Autodesk Inventor part; units mm, degrees
ref_plane "Work Plane1" through (-106.5, -37, 0) normal (1, 0, 0) x (0, 1, 0)
ref_plane "Work Plane2" through (-183, -37, 0) normal (1, 0, 0) x (0, 1, 0)
ref_plane "Work Plane3" through (-106.5, -37, -17.5) normal (0, -1, 0) x (1, 0, 0)
sketch "Sketch1" plane through (0, 0, 0) normal (0, 0, 1) x (1, 0, 0)
  line L0 (-183, -19.5) -> (-106.5, -19.5)
  line L1 (-106.5, -19.5) -> (-106.5, -54.5)
  line L2 (-106.5, -54.5) -> (-183, -54.5)
  line L3 (-183, -54.5) -> (-183, -19.5)
  line L4 (-194, -37) -> (-96, -37) construction
  line L5 (-183, -22) -> (-157.5, -22)
  line L6 (-157.5, -22) -> (-157.5, -37)
  line L7 (-157.5, -24.5) -> (-116.5, -24.5)
  line L8 (-116.5, -37) -> (-116.5, -22)
  line L9 (-116.5, -22) -> (-106.5, -22)
  line L10 (-183, -52) -> (-157.5, -52) construction
  line L11 (-157.5, -52) -> (-157.5, -37) construction
  line L12 (-157.5, -49.5) -> (-116.5, -49.5) construction
  line L13 (-116.5, -37) -> (-116.5, -52) construction
  line L14 (-116.5, -52) -> (-106.5, -52) construction
  line L15 (-183, -37) -> (-106.5, -37)
  point P0 (0, 0)
  dimension "d0" = 76.5
  dimension "d1" = 35
  dimension "d2" = 30
  dimension "d3" = 25.5
  dimension "d4" = 10
  dimension "d5" = 25
  dimension "d6" = 30
sketch "Sketch3" plane through (0, 0, 0) normal (1, 0, 0) x (0, 1, 0)
  point P0 (0, 0)
ref_plane "Work Plane1" through (-106.5, -37, 0) normal (1, 0, 0) x (0, 1, 0)
sketch "Sketch4" plane through (-106.5, -37, 0) normal (1, 0, 0) x (0, 1, 0)
  point P0 (37, 0)
sketch "Sketch5" plane through (-106.5, -37, 0) normal (1, 0, 0) x (0, 1, 0)
  line L0 (-17.5, 17.5) -> (17.5, 17.5)
  line L1 (17.5, 17.5) -> (17.5, -17.5)
  line L2 (17.5, -17.5) -> (-17.5, -17.5)
  line L3 (-17.5, -17.5) -> (-17.5, 17.5)
  line L4 (-17.5, 17.5) -> (17.5, -17.5) construction
  line L5 (17.5, 17.5) -> (-17.5, -17.5) construction
  point P0 (37, 0)
  point P1 (0, 0)
  dimension "d10" = 35
  dimension "d11" = 35
ref_plane "Work Plane2" through (-183, -37, 0) normal (1, 0, 0) x (0, 1, 0)
extrude "Extrusion1" add sketch "Sketch5" against normal up to surface (76.5 mm away)
revolve "Revolution2" cut sketch "Sketch1" angle 360 about axis through (-194, -37, 0) along (1, 0, 0) contours L5 L6 L15 L3 | L1 L15 L8 L9 | L6 L7 L8 L15
sketch "Sketch7" plane through (-106.5, -37, 0) normal (1, 0, 0) x (0, 0, -1)
  circle A0 centre (0, 0) radius 19.09
  line L0 (-17.5, -17.5) -> (17.5, -17.5)
  line L1 (-17.5, 17.5) -> (-17.5, -17.5)
  line L2 (17.5, -17.5) -> (-17.5, 17.5) construction
  circle A1 centre (13.4987, -13.4987) radius 1.5
  circle A2 centre (13.4987, 13.4987) radius 1.5
  circle A3 centre (-13.4987, 13.4987) radius 1.5
  circle A4 centre (-13.4987, -13.4987) radius 1.5
  point P0 (0, 37)
  dimension "d21" = 38.18
  dimension "d22" = 3
  dimension "d25" = 360
hole "Hole1" at (-106.5, -23.5013, -13.4987) at (-106.5, -23.5013, 13.4987) at (-106.5, -50.4987, 13.4987) at (-106.5, -50.4987, -13.4987) direction (-1, 0, 0) diameter 2.5 depth 7 tip angle 118 counterbore diameter 3 counterbore depth 5
sketch "Sketch8" plane through (-183, -54.5, -17.5) normal (-1, 0, 0) x (0, 0, 1)
  line L0 (17.5, -7) -> (17.5, 46)
  circle A0 centre (2.5, 30) radius 1.25
  line L1 (0, 35) -> (0, 0)
  line L2 (35, 35) -> (0, 35)
  circle A1 centre (32.5, 30) radius 1.25
  circle A2 centre (17.5, 17.5) radius 15
  circle A3 centre (17.5, 17.5) radius 15
  line L3 (5.3, 6.5) -> (5.3, 35)
  line L4 (0, 35) -> (35, 35)
  arc A4 (5.3, 6.5) -> (6.3, 5.5) centre (6.3, 6.5) ccw
  line L5 (17.5, 5.5) -> (6.3, 5.5)
  line L6 (29.7, 6.5) -> (29.7, 35)
  arc A5 (28.7, 5.5) -> (29.7, 6.5) centre (28.7, 6.5) ccw
  line L7 (17.5, 5.5) -> (28.7, 5.5)
  point P0 (17.5, 54.5)
  point P1 (17.5, 5.5)
  point P2 (5.3, 35)
  dimension "d34" = 2.5
  dimension "d35" = 2.5
  dimension "d36" = 5
  dimension "d38" = 1
  dimension "d39" = 29.5
  dimension "d40" = 24.4
extrude "Extrusion2" cut sketch "Sketch8" against normal blind 2.75 contours L5 A2 L3 L0 | L0 A2 L6 L7 | L5 A4 L3 A2 | A2 L6 A5 L7 | A2 L3 L2 L0 | L0 L2 L6 A2
hole "Hole2" at (-183, -24.5, -15) at (-183, -24.5, 15) direction (1, 0, 0) diameter 2 depth 5 tip angle 118 counterbore diameter 2.5 counterbore depth 4
ref_plane "Work Plane3" through (-106.5, -37, -17.5) normal (0, -1, 0) x (1, 0, 0)
sketch "Sketch9" plane through (-106.5, -37, -17.5) normal (0, -1, 0) x (1, 0, 0)
  point P0 (106.5, 17.5)
sketch "Sketch11" plane through (-106.5, -19.5, 17.5) normal (0, 1, 0) x (1, 0, 0)
  line L0 (-73.75, 5.3) -> (-76.5, 5.3)
  line L1 (-76.5, 0) -> (-76.5, 5.3)
  line L2 (0, 0) -> (-76.5, 0)
  line L3 (0, 35) -> (0, 0)
  line L4 (0, 35) -> (-76.5, 35)
  line L5 (-76.5, 29.7) -> (-76.5, 35)
  line L6 (-76.5, 29.7) -> (-73.75, 29.7)
  line L7 (-73.75, 29.7) -> (-73.75, 5.3)
  line L8 (28.2317, 17.5) -> (-103.7683, 17.5) construction
  circle A0 centre (-30, 17.5) radius 1.5
  circle A1 centre (-50, 17.5) radius 2.5
  point P0 (106.5, 17.5)
  point P1 (0, 17.5)
  dimension "d54" = 3
  dimension "d55" = 5
  dimension "d56" = 30
  dimension "d57" = 50
extrude "Extrusion3" cut sketch "Sketch11" against normal up to surface (35 mm away) contours A0
extrude "Extrusion4" cut sketch "Sketch11" against normal up to surface contours A1
sketch "Sketch12" plane through (-106.5, -54.5, -17.5) normal (0, 0, -1) x (-1, 0, 0)
  line L0 (76.5, 35) -> (76.5, 0)
  line L1 (0, 35) -> (76.5, 35)
  line L2 (0, 0) -> (0, 35)
  line L3 (0, 0) -> (76.5, 0)
  line L4 (-16, 17.5) -> (90, 17.5)
  circle A0 centre (15, 5) radius 1.5
  circle A1 centre (45, 5) radius 1.5
  circle A2 centre (15, 30) radius 1.5
  circle A3 centre (45, 30) radius 1.5
  point P0 (-106.5, 54.5)
  point P1 (0, 17.5)
  dimension "d62" = 3
  dimension "d63" = 15
  dimension "d64" = 5
  dimension "d67" = 30
hole "Hole3" at (-121.5, -24.5, -17.5) at (-151.5, -24.5, -17.5) at (-151.5, -49.5, -17.5) at (-121.5, -49.5, -17.5) direction (0, 0, 1) diameter 2.5 depth 7 tip angle 118 counterbore diameter 3 counterbore depth 5
ref_plane "Work Plane4" through (-106.5, -54.5, 0) normal (0, 0, -1) x (-1, 0, 0)
mirror "Mirror2" about plane through (-106.5, -54.5, 0) normal (0, 0, -1) of "Hole3"
chamfer "Chamfer3" distance 0.5 angle 45 4 edges at (-151.5, -51, -17.5) (-151.5, -26, -17.5) (-121.5, -51, -17.5) (-121.5, -26, -17.5) measured on face at (-172.9115, -40.8826, -17.5)
chamfer "Chamfer4" distance 0.5 angle 45 4 edges at (-151.5, -26, 17.5) (-151.5, -51, 17.5) (-121.5, -26, 17.5) (-121.5, -51, 17.5) measured on face at (-172.9115, -33.1174, 17.5)
chamfer "Chamfer5" distance 0.5 angle 45 4 edges at (-106.5, -50.4987, -11.9987) (-106.5, -23.5013, -11.9987) (-106.5, -50.4987, 14.9987) (-106.5, -23.5013, 14.9987) measured on face at (-106.5, -37.6027, 16.6302)
properties part number "shaft box"
For this review, take the finished solid that the model builds, in its own axes (mm). A direction names the side the tool comes from. Give positions to 0.01 mm unless a question says otherwise; leave off trailing zeros. Write each loop counter-clockwise with the first axis right and the second up, starting at its lowest first coordinate (ties: lowest second). Pieces come first, ordered by that corner, then holes. Notation, with made-up numbers: M 7,62.25 L 33,62.25 A20 cw 33,81.25 Z; hole C 32.25,57 d5. An arc over 180 degrees is marked long. Answer as a JSON object with one key per item and string values. Group by question number.
Item 1: Tool access review of faces 3 (the cylindrical face through (-178.49, -23.61, -14.54)), 4 (the cylindrical face through (-154.115, -22.09, -0.751)), 5 (the cylindrical face through (-120.013, -24.695, 14.718)), 6 (the cylindrical face through (-150.391, -23.923, -11.486)): name each direction out of +Z, -Z, +X, -X, +Y, -Y from which nothing blocks a thin tool from reaching the whole face with its end or side.
Item 2: Consider section B-B on y = -37. Write out the cut boundary in (x, z), plus the area to 4 significant figures.
Item 3: For probe 1 along Z at (x, y) = (-161, -43); probe 2 along Y at (x, z) = (-165.5, -0.5); probe 3 along X at (y, z) = (-22.9, 0), list the stretches that pass through material, from the lowest coordinate up. Write a range as [from, to].
Item 4: Draft analysis for pull direction Y (two halves, no side actions). For faces 1 (the cylindrical face through (-122.554, -23.828, -11.486)), 2 (the flat face through (-182, -47, -12.2)), state which applies: +Y half, -Y half, draft (parallel to the pull), parting line (faces both ways), or undercut.
Item 5: Consider section A-A on x = -136.5. Write out the cut boundary in (y, z), plus the area to 3 significant figures.
Item 6: For pin 1 Ø3.5 at (x, y) = (-151, -49.5) entering from +Z; pin 2 Ø4 at (y, z) = (-46, -4.5) entering from -X; pin 3 Ø2 at (x, y) = (-121.5, -49.5) entering from +Z; pin 4 Ø2.5 at (x, y) = (-152, -50) entering from -Z, all flat-tipped, find the tip position at first contact; note any pin that passes through.
Item 7: Consider section C-C on z = 0. Write out the cut boundary in (x, y), plus the area to 3 significant figures.
Item 8: Consider section D-D on z = -6. Write out the cut boundary in (x, y), plus the area to 3 significant figures.
Check result:
{
 "1": {"face 3": "-X", "face 4": "+Y", "face 5": "+Z", "face 6": "-Z"},
 "2": {"outline": "M -183,-17.5 L -106.5,-17.5 L -106.5,-15 L -116.5,-15 L -116.5,-12.5 L -157.5,-12.5 L -157.5,-15 L -183,-15 Z; M -183,15 L -157.5,15 L -157.5,12.5 L -116.5,12.5 L -116.5,15 L -106.5,15 L -106.5,17.5 L -183,17.5 Z", "area": "587.5 mm^2"},
 "3": {"probe 1": "z = [-17.5, -13.75], [13.75, 17.5]", "probe 2": "y = [-54.5, -51.99], [-22.01, -19.5]", "probe 3": "x = [-154, -138], [-135, -116.5]"},
 "4": {"face 1": "undercut", "face 2": "draft"},
 "5": {"outline": "M -54.5,-17.5 L -19.5,-17.5 L -19.5,-1.5 L -24.59,-1.5 A12.5 cw -49.41,-1.5 L -54.5,-1.5 Z; M -54.5,1.5 L -49.41,1.5 A12.5 cw -24.59,1.5 L -19.5,1.5 L -19.5,17.5 L -54.5,17.5 Z", "area": "704 mm^2"},
 "6": {"pin 1": "stops at z = 17.5", "pin 2": "passes through", "pin 3": "stops at z = 10.35", "pin 4": "stops at z = -17.46"},
 "7": {"outline": "M -183,-54.5 L -138,-54.5 L -138,-49.5 L -157.5,-49.5 L -157.5,-52 L -183,-52 Z; M -180.25,-22 L -159,-22 L -159,-19.5 L -180.25,-19.5 Z; M -154,-24.5 L -138,-24.5 L -138,-19.5 L -154,-19.5 Z; M -135,-54.5 L -106.5,-54.5 L -106.5,-52 L -116.5,-52 L -116.5,-49.5 L -135,-49.5 Z; M -135,-24.5 L -116.5,-24.5 L -116.5,-22 L -106.5,-22 L -106.5,-19.5 L -135,-19.5 Z", "area": "529 mm^2"},
 "8": {"outline": "M -183,-54.5 L -106.5,-54.5 L -106.5,-50.75 L -116.5,-50.75 L -116.5,-47.97 L -157.5,-47.97 L -157.5,-50.75 L -183,-50.75 Z; M -180.25,-23.25 L -157.5,-23.25 L -157.5,-26.03 L -116.5,-26.03 L -116.5,-23.25 L -106.5,-23.25 L -106.5,-19.5 L -180.25,-19.5 Z", "area": "792 mm^2"}
}
